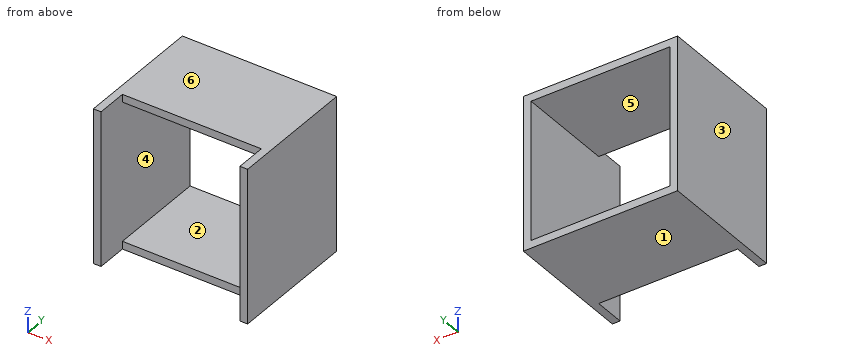
from build123d import *

# Parameters (mm, degrees)
SKETCH_1_W          = 60
SKETCH_1_H          = 60
EXTRUDE_1_DEPTH     = 50
SKETCH_2_W          = 54
SKETCH_2_H          = 54
CUT_EXTRUDE_2_DEPTH = 99.488578018
SKETCH_3_W          = 54
SKETCH_3_H          = 12
CUT_EXTRUDE_3_DEPTH = 99.488578018


with BuildPart() as part:
    # 草图1 → 凸台-拉伸1 (new body)
    with BuildSketch(Plane(origin=(0, 0, 0), x_dir=(1, 0, 0), z_dir=(0, 1, 0))):
        with Locations((30, 30)):
            Rectangle(SKETCH_1_W, SKETCH_1_H)
    extrude(amount=EXTRUDE_1_DEPTH)

    # 草图2 → 切除-拉伸2 (cut, through all)
    with BuildSketch(Plane(origin=(0, 0, 0), x_dir=(1, 0, 0), z_dir=(0, 1, 0))):
        with Locations((30, 30)):
            Rectangle(SKETCH_2_W, SKETCH_2_H)
    extrude(amount=CUT_EXTRUDE_2_DEPTH, mode=Mode.SUBTRACT)

    # 草图3 → 切除-拉伸3 (cut, through all)
    with BuildSketch(Plane.XY):
        with Locations((30, 6)):
            Rectangle(SKETCH_3_W, SKETCH_3_H)
    extrude(amount=-CUT_EXTRUDE_3_DEPTH, mode=Mode.SUBTRACT)


solid = part.part
Work out the finished part from the listing and answer in its coordinate system (mm). Face numbers are marked on the shaded views. A direction names the side the tool comes from. Coordinates: 2 decimals unless noted, no trailing zeros. Write each loop counter-clockwise with the first axis right and the second up, starting at its lowest first coordinate (ties: lowest second). Pieces come first, ordered by that corner, then holes. Notation, with made-up numbers: M -23.5,2 L 14.5,2 A23 ccw 14.5,26 Z; hole C 65.25,9 d8. An arc over 180 degrees is marked long. Answer as CSV lines item,"result". Start each with the question number.
Item 1: Section B-B on x = 32.5 is taken. Write down the section's boundary in (y, z).
Item 2: Section C-C on y = 33.5 is taken. Write down the section's boundary in (x, z).
Item 3: Consider L1, parallel to X at y = 44, z = -46; L2, parallel to Z at x = 42, y = 32. Determine where each line is inside the solid, lowest interval first.
Item 4: Section A-A on z = -9.5 is taken. Write down the section's boundary in (x, y), and give its area (3 significant figures).
Item 5: A tool of negligible diameter and unlimited length cuts with its end or side. For the marked faces 5 and 6, from which of +Z, -Z, +X, -X, +Y, -Y can it reach the whole face along a straight path? Write none if from no direction.
Item 6: Determine the mould class of the marked faces 1, 2, 3 and 4 for opening direction Z: released by +Z, released by -Z, zero draft, split by the parting line, or undercut.
Item 7: Flat-ended cylindrical pins translate along their axes: P1, Ø1.5, axis at x = 25.5, z = -58, coming from the -Y side; P2, Ø11.5, axis at x = 17, y = 30, coming from the +Z side. Find the tip coordinate at first contact, or state that the pin passes through.
Checks:
1,outline,"M 12,-60 L 50,-60 L 50,-57 L 12,-57 Z; M 12,-3 L 50,-3 L 50,0 L 12,0 Z"
2,outline,"M 0,-60 L 60,-60 L 60,0 L 0,0 Z; hole M 3,-57 L 57,-57 L 57,-3 L 3,-3 Z"
3,L1,"x = 0 to 3, 57 to 60"
3,L2,"z = -60 to -57, -3 to 0"
4,outline,"M 0,0 L 3,0 L 3,50 L 0,50 Z; M 57,0 L 60,0 L 60,50 L 57,50 Z"
4,area,"300 mm²"
5,face 5,"+Y, -Y"
5,face 6,"+Z, +X, -X, +Y, -Y"
6,face 1,"released by -Z"
6,face 2,"undercut"
6,face 3,"zero draft"
6,face 4,"undercut"
7,P1,"stops at y = 12"
7,P2,"stops at z = 0"
